```python
from build123d import *

# Parameters (mm, degrees)
SKETCH1_R           = 3.25
BOSS_EXTRUDE1_DEPTH = 7.018
SKETCH6_R           = 4.7
BOSS_EXTRUDE2_DEPTH = 10
BOSS_EXTRUDE3_DEPTH = 1
FILLET1_R           = 0.75
BOSS_EXTRUDE4_DEPTH = 2


with BuildPart() as part:
    # Sketch1 → Boss-Extrude1 (new body)
    with BuildSketch(Plane(origin=(0, 0, 0), x_dir=(1, 0, 0), z_dir=(0, 1, 0))):
        Circle(SKETCH1_R)
    extrude(amount=BOSS_EXTRUDE1_DEPTH)

    # Sketch6 → Boss-Extrude2 (add)
    with BuildSketch(Plane(origin=(0, 7.018, 0), x_dir=(1, 0, 0), z_dir=(0, 1, 0))):
        Circle(SKETCH6_R)
    extrude(amount=BOSS_EXTRUDE2_DEPTH)

    # Sketch8 → Boss-Extrude3 (add)
    with BuildSketch(Plane(origin=(0, 17.018, 0), x_dir=(1, 0, 0), z_dir=(0, 1, 0))):
        Polygon((0.4, 3.75), (-0.4, 3.75), (-0.4, 0.4), (-3.75, 0.4), (-3.75, -0.4), (-0.4, -0.4), (-0.4, -3.75), (0.4, -3.75), (0.4, -0.4), (3.75, -0.4), (3.75, 0.4), (0.4, 0.4), align=None)
    extrude(amount=BOSS_EXTRUDE3_DEPTH)

    # Fillet1
    fillet1_edges = [part.edges().sort_by_distance(p)[0] for p in [
        (-4.7, 17.018, 0),
    ]]
    fillet(fillet1_edges, radius=FILLET1_R)

    # Sketch10 → Boss-Extrude4 (add)
    with BuildSketch(Plane.XZ.offset(-7.018)):
        with BuildLine():
            Line((4.169549594, 2.169068046), (6.132310873, 2.694988345))
            Line((6.132310873, 2.694988345), (6.658231172, 0.732227066))
            Line((6.658231172, 0.732227066), (4.695469893, 0.206306767))
            ThreePointArc((4.695469893, 0.206306767), (4.539851384, 1.216449512), (4.169549594, 2.169068046))
        make_face()
        with BuildLine():
            Line((-4.677844754, 0.45581625), (-6.640606033, -0.07010405))
            Line((-6.640606033, -0.07010405), (-5.785985547, -3.259591128))
            Line((-5.785985547, -3.259591128), (-3.823224268, -2.733670829))
            ThreePointArc((-3.823224268, -2.733670829), (-4.539851384, -1.216449512), (-4.677844754, 0.45581625))
        make_face()
    extrude(amount=-BOSS_EXTRUDE4_DEPTH)


solid = part.part
```
Geometry check sheet. Reference: the model listing, model coordinates, mm. A direction names the side the tool comes from. Round coordinates to 2 decimals unless told otherwise and drop trailing zeros. Loops run counter-clockwise (first coordinate to the right, second up) from the corner with the lowest first, then second, coordinate; pieces in that order, holes last. Notation, with made-up numbers: (63, 53.5) - (70, 53.5) arc R34 ccw to (70, 89.5) - close; hole circle Ø5 at (49.25, -40). An arc over 180 degrees is marked (long way). Use a Markdown table: item, result.
Q1. Go/stop test with flat-tipped pins: P1, Ø1.2, axis at x = 5.5, z = 1, coming from the +Y side; P2, Ø0.5, axis at y = 17.5, z = -2, coming from the -X side; P3, Ø0.8, axis at x = 2.5, y = 17.5, coming from the -Z side. Record where each tip stops, or that it passes through.
Solutions:
| item | result |
|---|---|
| P1 | stops at y = 9.02 |
| P2 | stops at x = -0.4 |
| P3 | stops at z = -0.4 |
Q2. Cross-section at A-A on x = 0. Record the cut outline in (y, z), plus the area to 3 significant figures.
Solutions:
| item | result |
|---|---|
| outline | (0, -3.25) - (7.02, -3.25) - (7.02, -4.7) - (16.27, -4.7) arc R0.75 ccw to (17.02, -3.95) - (17.02, -3.75) - (18.02, -3.75) - (18.02, 3.75) - (17.02, 3.75) - (17.02, 3.95) arc R0.75 ccw to (16.27, 4.7) - (7.02, 4.7) - (7.02, 3.25) - (0, 3.25) - close |
| area | 147 mm2 |
Q3. Cross-section at C-C on y = 5.5. Record the cut outline in (x, z), plus the area to 3 significant figures.
Solutions:
| item | result |
|---|---|
| outline | circle Ø6.5 at (0, 0) |
| area | 33.2 mm2 |
Q4. Material ranges on line 1 (Y direction, x = -2, z = 1); line 2 (X direction, y = 16, z = 0); line 3 (Z direction, x = -2.75, y = 9), recorded low to high.
Solutions:
| item | result |
|---|---|
| line 1 | y = 0 to 17.02 |
| line 2 | x = -4.7 to 4.7 |
| line 3 | z = -3.81 to 3.81 |
Q5. Access from +Z, -Z, +X, -X, +Y, -Y to the whole of each face (thin tool, end or side, straight path). Record for faces 4 (the flat face through (-4.82, 8, -3)), 5 (the flat face through (0.4, 17.5, -2.1)), 6 (the flat face through (-2.1, 17.5, -0.4)).
Solutions:
| item | result |
|---|---|
| face 4 | -Z, +Y, -Y |
| face 5 | -Z, +X, +Y |
| face 6 | -Z, -X, +Y |
Q6. Cross-section at B-B on y = 15.5. Record the cut outline in (x, z), plus the area to 3 significant figures.
Solutions:
| item | result |
|---|---|
| outline | circle Ø9.4 at (0, 0) |
| area | 69.4 mm2 |
Q7. Draft check along X on faces 1 (the flat face through (-2.1, 17.5, 0.4)), 2 (the flat face through (5.691, 8.004, 0.473)), 3 (the flat face through (5.14, 8, 2.43)). Enter one of: released by +X, released by -X, zero draft, split by the parting line, or undercut.
Solutions:
| item | result |
|---|---|
| face 1 | zero draft |
| face 2 | released by +X |
| face 3 | undercut |
Q8. Cross-section at D-D on x = 5.5. Record the cut outline in (y, z), plus the area to 3 significant figures.
Solutions:
| item | result |
|---|---|
| outline | (7.02, 0.42) - (9.02, 0.42) - (9.02, 2.53) - (7.02, 2.53) - close |
| area | 4.21 mm2 |
